Print and shaded views of the part. All mm, measured from the part's lowest x, y and z. Round coordinates to 2 decimals unless told otherwise and drop trailing zeros. Loops run counter-clockwise (first coordinate to the right, second up) from the corner with the lowest first, then second, coordinate; pieces in that order, holes last. Notation, with made-up numbers: (75.5, 54.25) -> (108.5, 54.25) arc R24 cw to (108.5, 81.25) -> close; hole circle Ø10 at (8.25, 55). An arc over 180 degrees is marked (long way). Answer as CSV lines item,"result".
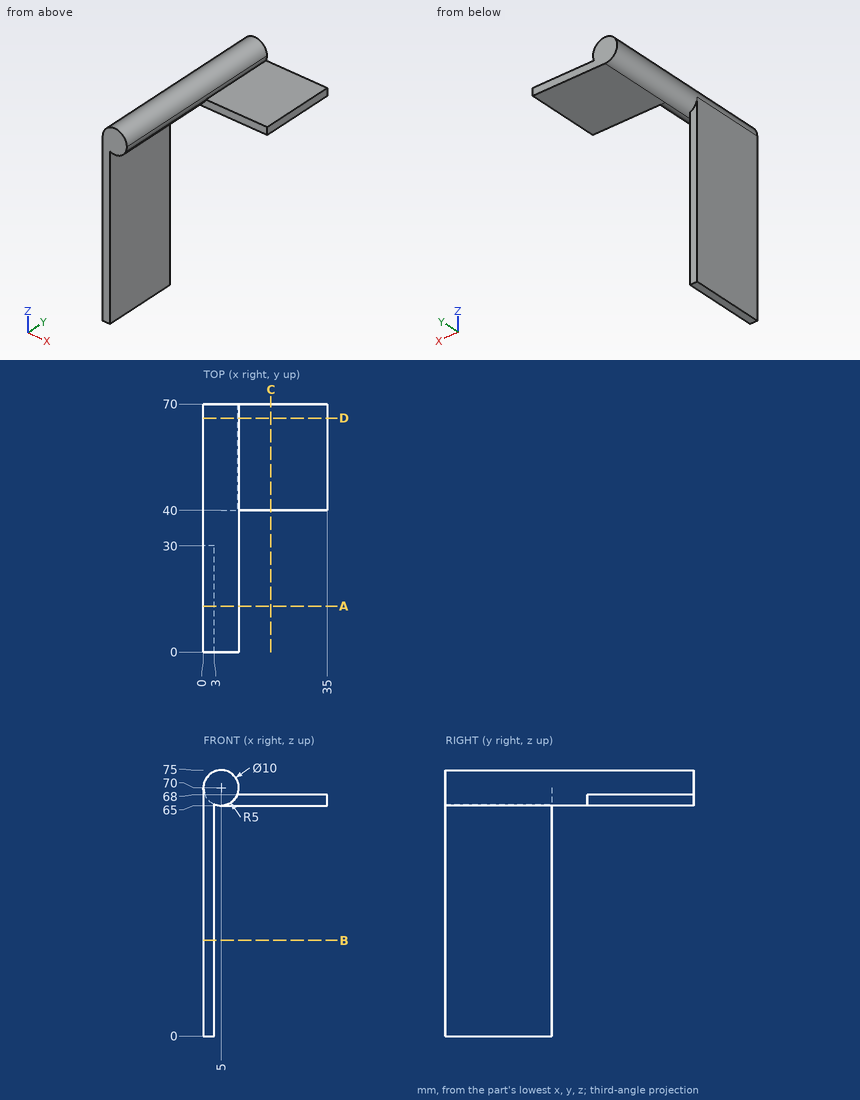
Q1. Saw through at B-B, the plane z = 27. Write the cut outline in (x, y), then the cut area to 3 significant figures.
Geometry results:
outline,"(0, 0) -> (3, 0) -> (3, 30) -> (0, 30) -> close"
area,"90.0 mm2"
Q2. Drill centre lines: line 1 along Z through (x, y) = (22.5, 52.5); line 2 along X through (y, z) = (6.5, 36.5); line 3 along X through (y, z) = (26.5, 68). Where is each one in solid material? Low to high.
Geometry results:
line 1,"65 to 68"
line 2,"0 to 3"
line 3,"0 to 9.58"
Q3. Drop flat-ended pins along their axis: P1, Ø2, axis at x = 6, y = 61, coming from the -Z side; P2, Ø5, axis at x = 9.5, y = 26, coming from the +Z side; P3, Ø9, axis at y = 14.5, z = 39.5, coming from the +X side. Give the stop position or say it passes through.
Geometry results:
P1,"z = 65"
P2,"z = 74.58"
P3,"x = 3"
Q4. Saw through at C-C, the plane x = 19. Write the cut outline in (y, z).
Geometry results:
outline,"(40, 65) -> (70, 65) -> (70, 68) -> (40, 68) -> close"
Q5. Saw through at A-A, the plane y = 13. Write the cut outline in (x, z).
Geometry results:
outline,"(0, 0) -> (3, 0) -> (3, 65.42) arc R5 ccw (long way) to (0, 70) -> close"
Q6. Saw through at D-D, the plane y = 66. Write the cut outline in (x, z), then the cut area to 3 significant figures.
Geometry results:
outline,"(5, 65) -> (35, 65) -> (35, 68) -> (9.58, 68) arc R5 ccw (long way) to start"
area,"159 mm2"
